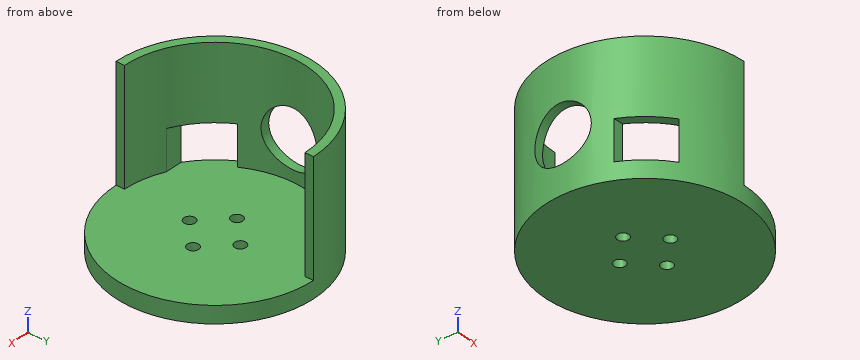
```python
from build123d import *

# Parameters (mm, degrees)
SKIZZE3_R                       = 17.5
SKIZZE3_R_2                     = 16
AUFSATZ_LINEAR_AUSTRAGEN3_DEPTH = 20
SKIZZE4_R                       = 17.5
AUFSATZ_LINEAR_AUSTRAGEN4_DEPTH = 3
SKIZZE5_R                       = 5
SCHNITT_LINEAR_AUSTRAGEN1_DEPTH = 40
SKIZZE6_R                       = 1
SCHNITT_LINEAR_AUSTRAGEN2_DEPTH = 10
SKIZZE7_W                       = 31.87732214
SKIZZE7_H                       = 34.999785002
SCHNITT_LINEAR_AUSTRAGEN3_DEPTH = 30
SKIZZE8_W                       = 7
SKIZZE8_H                       = 6.5
SCHNITT_LINEAR_AUSTRAGEN4_DEPTH = 30


with BuildPart() as part:
    # Skizze3 → Aufsatz-Linear austragen3 (new body)
    with BuildSketch(Plane.XY):
        Circle(SKIZZE3_R)
        Circle(SKIZZE3_R_2, mode=Mode.SUBTRACT)
    extrude(amount=AUFSATZ_LINEAR_AUSTRAGEN3_DEPTH)

    # Skizze4 → Aufsatz-Linear austragen4 (add)
    with BuildSketch(Plane.XY):
        Circle(SKIZZE4_R)
    extrude(amount=-AUFSATZ_LINEAR_AUSTRAGEN4_DEPTH)

    # Skizze5 → Schnitt-Linear austragen1 (cut)
    with BuildSketch(Plane(origin=(0, 0, 0), x_dir=(0, 0, -1), z_dir=(1, 0, 0))):
        with Locations((-7, 0)):
            Circle(SKIZZE5_R)
    extrude(amount=-SCHNITT_LINEAR_AUSTRAGEN1_DEPTH, mode=Mode.SUBTRACT)

    # Skizze6 → Schnitt-Linear austragen2 (cut)
    with BuildSketch(Plane(origin=(0, 0, -3), x_dir=(-1, 0, 0), z_dir=(0, 0, -1))):
        with Locations((-4.5, 0)):
            Circle(SKIZZE6_R)
        with Locations((0, 4.5)):
            Circle(SKIZZE6_R)
        with Locations((4.5, 0)):
            Circle(SKIZZE6_R)
        with Locations((0, -4.5)):
            Circle(SKIZZE6_R)
    extrude(amount=-SCHNITT_LINEAR_AUSTRAGEN2_DEPTH, mode=Mode.SUBTRACT)

    # Skizze7 → Schnitt-Linear austragen3 (cut)
    with BuildSketch(Plane.XY):
        with Locations((16, 0)):
            Rectangle(SKIZZE7_W, SKIZZE7_H)
    extrude(amount=SCHNITT_LINEAR_AUSTRAGEN3_DEPTH, mode=Mode.SUBTRACT)

    # Skizze8 → Schnitt-Linear austragen4 (cut)
    with BuildSketch(Plane(origin=(0, 0, 0), x_dir=(0, 0, -1), z_dir=(1, 0, 0))):
        with Locations((-3.5, -11.25)):
            Rectangle(SKIZZE8_W, SKIZZE8_H)
    extrude(amount=-SCHNITT_LINEAR_AUSTRAGEN4_DEPTH, mode=Mode.SUBTRACT)


solid = part.part
```
For this review, take the finished solid that the model builds, in its own axes (mm). Round coordinates to 2 decimals unless told otherwise and drop trailing zeros. Write each loop counter-clockwise with the first axis right and the second up, starting at its lowest first coordinate (ties: lowest second). Pieces come first, ordered by that corner, then holes. Notation, with made-up numbers: (17, -11.5) -> (23, -11.5) arc R26 ccw to (23, 12.5) -> close; hole circle Ø11 at (39.25, 32). An arc over 180 degrees is marked (long way). One line per question, with ' | ' between items. Start each with the question number.
(1) Add section C-C, the plane x = -4.5. Write out the cut boundary in (y, z), plus the area to 3 significant figures.
(2) Add section A-A, the plane y = 0. Write out the cut boundary in (x, z), plus the area to 3 significant figures.
(3) Insertion check: P1, Ø8, axis at y = 6.5, z = -0.5, coming from the -X side; P2, Ø11.5, axis at y = 0, z = 7, coming from the -X side; P3, Ø1.5, axis at x = 11.5, y = 2.5, coming from the +Z side; P4, Ø0.8, axis at y = -16.5, z = 10, coming from the +X side. Each pin has a flat end and moves straight along its axis. Give the tip position at first contact, or say it passes through.
(4) Add section B-B, the plane z = 0.5. Write out the cut boundary in (x, y).
(5) For line 1 along Y through (x, z) = (0, -0.7); line 2 along Z through (x, y) = (-16.5, 0); line 3 along Z through (x, y) = (8.5, 13), list the stretches that pass through material, from the lowest coordinate up. Write a range as from..to.
(6) Add section D-D, the plane z = 3. Write out the cut boundary in (x, y).
Answer list:
1) outline: (-16.91, -3) -> (-1, -3) -> (-1, 0) -> (-15.35, 0) -> (-15.35, 20) -> (-16.91, 20) -> close; (1, -3) -> (16.91, -3) -> (16.91, 20) -> (15.35, 20) -> (15.35, 0) -> (1, 0) -> close | area: 158 mm²
2) outline: (-17.5, -3) -> (-5.5, -3) -> (-5.5, 0) -> (-16, 0) -> (-16, 2) -> (-17.5, 2) -> close; (-17.5, 12) -> (-16, 12) -> (-16, 20) -> (-17.5, 20) -> close; (-3.5, -3) -> (3.5, -3) -> (3.5, 0) -> (-3.5, 0) -> close; (5.5, -3) -> (17.5, -3) -> (17.5, 0) -> (5.5, 0) -> close | area: 108 mm²
3) P1: x = -17.32 | P2: x = -17.5 | P3: z = 0 | P4: x = 0.06
4) outline: (-15.56, -8) -> (-13.86, -8) arc R16 cw to (0.06, 16) -> (0.06, 17.5) arc R17.5 ccw to start; (-9.8, -14.5) arc R17.5 ccw to (0.06, -17.5) -> (0.06, -16) arc R16 cw to (-6.76, -14.5) -> close
5) line 1: -17.5..-5.5, -3.5..3.5, 5.5..17.5 | line 2: -3..2, 12..20 | line 3: -3..0
6) outline: (-17.24, -3) arc R17.5 ccw to (-15.56, -8) -> (-13.86, -8) arc R16 cw to (-15.72, -3) -> close; (-17.24, 3) -> (-15.72, 3) arc R16 cw to (0.06, 16) -> (0.06, 17.5) arc R17.5 ccw to start; (-9.8, -14.5) arc R17.5 ccw to (0.06, -17.5) -> (0.06, -16) arc R16 cw to (-6.76, -14.5) -> close
